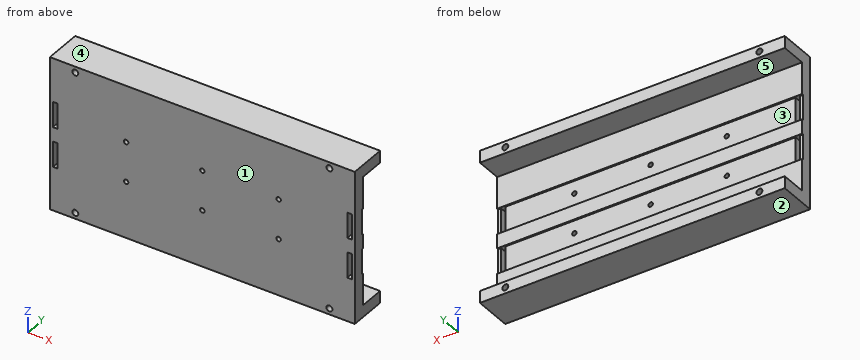
from build123d import *

# Parameters (mm, degrees)
SKETCH1_W           = 102
SKETCH1_H           = 51
BOSS_EXTRUDE2_DEPTH = 4
SKETCH2_W           = 102
SKETCH2_H           = 4
BOSS_EXTRUDE3_DEPTH = 8.6
SKETCH3_W           = 102
SKETCH3_H           = 8.5
CUT_EXTRUDE2_DEPTH  = 0.5
SKETCH4_R           = 0.75
SKETCH4_W           = 1.5
SKETCH4_H           = 8.5
CUT_EXTRUDE4_DEPTH  = 10
SKETCH6_R           = 1
CUT_EXTRUDE5_DEPTH  = 15


with BuildPart() as part:
    # Sketch1 → Boss-Extrude2 (new body)
    with BuildSketch(Plane(origin=(0, 0, 0), x_dir=(1, 0, 0), z_dir=(0, 1, 0))):
        with Locations((51, 25.5)):
            Rectangle(SKETCH1_W, SKETCH1_H)
    extrude(amount=BOSS_EXTRUDE2_DEPTH)

    # Sketch2 → Boss-Extrude3 (add)
    with BuildSketch(Plane(origin=(0, 4, 0), x_dir=(1, 0, 0), z_dir=(0, 1, 0))):
        with Locations((51, 49)):
            Rectangle(SKETCH2_W, SKETCH2_H)
        with Locations((51, 2)):
            Rectangle(SKETCH2_W, SKETCH2_H)
    extrude(amount=BOSS_EXTRUDE3_DEPTH)

    # Sketch3 → Cut-Extrude2 (cut)
    with BuildSketch(Plane(origin=(0, 4, 0), x_dir=(1, 0, 0), z_dir=(0, 1, 0))):
        with Locations((51, 18.85)):
            Rectangle(SKETCH3_W, SKETCH3_H)
        with Locations((51, 32.15)):
            Rectangle(SKETCH3_W, SKETCH3_H)
    extrude(amount=-CUT_EXTRUDE2_DEPTH, mode=Mode.SUBTRACT)

    # Sketch4 → Cut-Extrude4 (cut)
    with BuildSketch(Plane(origin=(0, 3.5, 0), x_dir=(1, 0, 0), z_dir=(0, 1, 0))):
        with Locations(Location((51, 18.85, 0), (0, 0, 270))):
            Circle(SKETCH4_R)
        with Locations(Location((76.5, 18.85, 0), (0, 0, 270))):
            Circle(SKETCH4_R)
        with Locations(Location((25.5, 18.85, 0), (0, 0, 270))):
            Circle(SKETCH4_R)
        with Locations(Location((76.5, 32.15, 0), (0, 0, 270))):
            Circle(SKETCH4_R)
        with Locations(Location((51, 32.15, 0), (0, 0, 270))):
            Circle(SKETCH4_R)
        with Locations(Location((25.5, 32.15, 0), (0, 0, 270))):
            Circle(SKETCH4_R)
        with Locations((100.25, 18.85)):
            Rectangle(SKETCH4_W, SKETCH4_H)
        with Locations((100.25, 32.15)):
            Rectangle(SKETCH4_W, SKETCH4_H)
        with Locations((1.75, 18.85)):
            Rectangle(SKETCH4_W, SKETCH4_H)
        with Locations((1.75, 32.15)):
            Rectangle(SKETCH4_W, SKETCH4_H)
    extrude(amount=-CUT_EXTRUDE4_DEPTH, mode=Mode.SUBTRACT)

    # Sketch6 → Cut-Extrude5 (cut)
    with BuildSketch(Plane(origin=(0, 12.6, 0), x_dir=(1, 0, 0), z_dir=(0, 1, 0))):
        with Locations(Location((93.5, 2, 0), (0, 0, 270))):
            Circle(SKETCH6_R)
        with Locations(Location((8.5, 2, 0), (0, 0, 270))):
            Circle(SKETCH6_R)
        with Locations(Location((93.5, 49, 0), (0, 0, 270))):
            Circle(SKETCH6_R)
        with Locations(Location((8.5, 49, 0), (0, 0, 270))):
            Circle(SKETCH6_R)
    extrude(amount=-CUT_EXTRUDE5_DEPTH, mode=Mode.SUBTRACT)


solid = part.part
For this review, take the finished solid that the model builds, in its own axes (mm). Face numbers are marked on the shaded views. A direction names the side the tool comes from. Coordinates: 2 decimals unless noted, no trailing zeros. Order: outer loops, then holes, each group sorted by start corner. A loop starts at its lowest first (then second) coordinate and runs counter-clockwise, first axis right, second up. Notation, with made-up numbers: (82, 52) - (121, 52) arc R20 ccw to (121, 85) - close; hole circle Ø11 at (52.5, -31). An arc over 180 degrees is marked (long way). Answer as CSV lines item,"result". Start each with the question number.
1) Add section A-A (y = 6.5). State the section outline as (x, z) points.
2) Machinability: for the marked faces 4 and 5, which of the approach directions +Z, -Z, +X, -X, +Y, -Y give a long, thin tool a straight path to every point of the face, cutting with its end or side? Answer none if there is none.
3) Add section B-B (z = -2). State the section outline as (x, y) points, then the cut area to 3 significant figures.
4) Add section C-C (x = 93.5). State the section outline as (y, z) points, then the cut area to 3 significant figures.
5) To check wall thickness, follow line 1 along X through (y, z) = (1.2, -18.85); line 2 along X through (y, z) = (2.5, -35); line 3 along X through (y, z) = (6.5, -49). State the ranges of each line that lie inside material, in increasing order. Write a range as [from, to].
6) Draft analysis for pull direction Z (two halves, no side actions). For the marked faces 1, 2 and 3, state which applies: +Z half, -Z half, draft (parallel to the pull), parting line (faces both ways), or undercut.
7) Insertion check: P1, Ø0.9, axis at x = 25.5, z = -18.85, coming from the +Y side; P2, Ø0.8, axis at x = 0.5, z = -34, coming from the +Y side; P3, Ø5.5, axis at x = 72.5, z = -25, coming from the +Y side. Each pin has a flat end and moves straight along its axis. Give the tip position at first contact, or say it passes through.
8) Add section D-D (x = 56.5). State the section outline as (y, z) points.
Result:
1,outline,"(0, -51) - (102, -51) - (102, -47) - (0, -47) - close; (0, -4) - (102, -4) - (102, 0) - (0, 0) - close; hole circle Ø2 at (8.5, -49); hole circle Ø2 at (8.5, -2); hole circle Ø2 at (93.5, -49); hole circle Ø2 at (93.5, -2)"
2,face 4,"+Z, +X, -X, +Y, -Y"
2,face 5,"+X, -X, +Y"
3,outline,"(0, 0) - (7.5, 0) - (7.5, 12.6) - (0, 12.6) - close; (9.5, 0) - (92.5, 0) - (92.5, 12.6) - (9.5, 12.6) - close; (94.5, 0) - (102, 0) - (102, 12.6) - (94.5, 12.6) - close"
3,area,"1,230 mm^2"
4,outline,"(0, -51) - (12.6, -51) - (12.6, -50) - (0, -50) - close; (0, -48) - (12.6, -48) - (12.6, -47) - (4, -47) - (4, -36.4) - (3.5, -36.4) - (3.5, -27.9) - (4, -27.9) - (4, -23.1) - (3.5, -23.1) - (3.5, -14.6) - (4, -14.6) - (4, -4) - (12.6, -4) - (12.6, -3) - (0, -3) - close; (0, -1) - (12.6, -1) - (12.6, 0) - (0, 0) - close"
4,area,"214 mm^2"
5,line 1,"[0, 1], [2.5, 24.75], [26.25, 50.25], [51.75, 75.75], [77.25, 99.5], [101, 102]"
5,line 2,"[0, 1], [2.5, 99.5], [101, 102]"
5,line 3,"[0, 7.5], [9.5, 92.5], [94.5, 102]"
6,face 1,"draft"
6,face 2,"-Z half"
6,face 3,"undercut"
7,P1,"through"
7,P2,"y = 3.5"
7,P3,"y = 4"
8,outline,"(0, -51) - (12.6, -51) - (12.6, -47) - (4, -47) - (4, -36.4) - (3.5, -36.4) - (3.5, -27.9) - (4, -27.9) - (4, -23.1) - (3.5, -23.1) - (3.5, -14.6) - (4, -14.6) - (4, -4) - (12.6, -4) - (12.6, 0) - (0, 0) - close"
